from build123d import *

# Parameters (mm, degrees)
SKETCH1_W           = 88
SKETCH1_H           = 88
BOSS_EXTRUDE1_DEPTH = 2
FILLET1_R           = 2
SKETCH3_R           = 1.85
CUT_EXTRUDE1_DEPTH  = 10
SKETCH4_R           = 2.5
CUT_EXTRUDE2_DEPTH  = 10


with BuildPart() as part:
    # Sketch1 → Boss-Extrude1 (new body)
    with BuildSketch(Plane(origin=(0, 0, 0), x_dir=(1, 0, 0), z_dir=(0, 1, 0))):
        Rectangle(SKETCH1_W, SKETCH1_H)
    extrude(amount=BOSS_EXTRUDE1_DEPTH)

    # Fillet1
    fillet1_edges = [part.edges().sort_by_distance(p)[0] for p in [
        (-44, 1, -44),
        (44, 1, -44),
        (44, 1, 44),
        (-44, 1, 44),
    ]]
    fillet(fillet1_edges, radius=FILLET1_R)

    # Sketch3 → Cut-Extrude1 (cut)
    with BuildSketch(Plane(origin=(0, 2, 0), x_dir=(1, 0, 0), z_dir=(0, 1, 0))):
        with Locations(Location((-25, 38.82, 0), (0, 0, 270))):
            Circle(SKETCH3_R)
        with Locations(Location((25, 38.82, 0), (0, 0, 270))):
            Circle(SKETCH3_R)
        with Locations(Location((-25, -38.82, 0), (0, 0, 270))):
            Circle(SKETCH3_R)
        with Locations(Location((25, -38.82, 0), (0, 0, 270))):
            Circle(SKETCH3_R)
    extrude(amount=-CUT_EXTRUDE1_DEPTH, mode=Mode.SUBTRACT)

    # Sketch4 → Cut-Extrude2 (cut)
    with BuildSketch(Plane(origin=(0, 2, 0), x_dir=(1, 0, 0), z_dir=(0, 1, 0))):
        with Locations(Location((-12.5, 10, 0), (0, 0, 270))):
            Circle(SKETCH4_R)
        with Locations(Location((-12.5, -10, 0), (0, 0, 270))):
            Circle(SKETCH4_R)
        with Locations(Location((12.5, -10, 0), (0, 0, 270))):
            Circle(SKETCH4_R)
        with Locations(Location((12.5, 10, 0), (0, 0, 270))):
            Circle(SKETCH4_R)
    extrude(amount=-CUT_EXTRUDE2_DEPTH, mode=Mode.SUBTRACT)


solid = part.part
Check sheet for the modelled part. Datum: model origin and axes. Units: mm. Round coordinates to 2 decimals unless told otherwise and drop trailing zeros. Write each loop counter-clockwise with the first axis right and the second up, starting at its lowest first coordinate (ties: lowest second). Pieces come first, ordered by that corner, then holes. Notation, with made-up numbers: (-35.75, 82.25) - (-6.75, 82.25) arc R32 ccw to (-6.75, 120.25) - close; hole circle Ø10 at (-2, -34). An arc over 180 degrees is marked (long way). Return JSON: item names as keys, results as strings.
Q1. Cross-section at C-C (z = 38.82). Record the boundary of the cut face in (x, y).
Returned:
{"outline": "(-44, 0) - (-26.85, 0) - (-26.85, 2) - (-44, 2) - close; (-23.15, 0) - (23.15, 0) - (23.15, 2) - (-23.15, 2) - close; (26.85, 0) - (44, 0) - (44, 2) - (26.85, 2) - close"}
Q2. Depth check by flat-ended pin: P1, Ø4.5, axis at x = 12.5, z = -10, coming from the +Y side. Enter the tip coordinate at first touch or a pass-through.
Returned:
{"P1": "passes through"}
Q3. Cross-section at B-B (y = 1). Give the number of separate pieces and of enclosed holes in the cut face, then the cut area to 3 significant figures.
Returned:
{"separate pieces": "1", "enclosed holes": "8", "area": "7,620 mm²"}
Q4. Scan lines: L1, parallel to X at y = 0.9, z = -38.82; L2, parallel to X at y = 1.2, z = 10; L3, parallel to Z at x = -24.5, y = 0.35. Record each from-to range of solid material in increasing order. Write a range as from..to.
Returned:
{"L1": "x = -44..-26.85, -23.15..23.15, 26.85..44", "L2": "x = -44..-15, -10..10, 15..44", "L3": "z = -44..-40.6, -37.04..37.04, 40.6..44"}
Q5. Cross-section at A-A (x = 25). Record the boundary of the cut face in (y, z).
Returned:
{"outline": "(0, -44) - (2, -44) - (2, -40.67) - (0, -40.67) - close; (0, -36.97) - (2, -36.97) - (2, 36.97) - (0, 36.97) - close; (0, 40.67) - (2, 40.67) - (2, 44) - (0, 44) - close"}
Q6. Draft check along Z on faces 1 (the cylindrical face through (26.834, 1.014, -39.061)), 2 (the cylindrical face through (43.4, 1.01, 43.43)), 3 (the flat face through (-1, 0, -1)). Enter one of: released by +Z, released by -Z, zero draft, split by the parting line, or undercut.
Returned:
{"face 1": "undercut", "face 2": "released by +Z", "face 3": "zero draft"}
